Verification items for the finished model (mm, model axes). A direction names the side the tool comes from. Give positions to 0.01 mm unless a question says otherwise; leave off trailing zeros. Order: outer loops, then holes, each group sorted by start corner. A loop starts at its lowest first (then second) coordinate and runs counter-clockwise, first axis right, second up. Notation, with made-up numbers: (14, 73.25) - (19, 73.25) arc R13 cw to (19, 95.25) - close; hole circle Ø10 at (-40, 83). An arc over 180 degrees is marked (long way). Answer as a JSON object with one key per item and string values.
Autodesk Inventor part; units mm, degrees
ref_plane "YZ Plane" through (0, 0, 0) normal (1, 0, 0) x (0, 1, 0)
ref_plane "XZ Plane" through (0, 0, 0) normal (0, 1, 0) x (-1, 0, 0)
ref_plane "XY Plane" through (0, 0, 0) normal (0, 0, 1) x (1, 0, 0)
sketch "Sketch1" plane through (0, 0, 0) normal (0, 1, 0) x (-1, 0, 0)
  arc A0 (0, -16) -> (0, 16) centre (0, 0) ccw
  arc A1 (0, -11.5) -> (0, 11.5) centre (0, 0) ccw
  line L0 (0, 16) -> (0, 11.5)
  line L1 (0, -11.5) -> (0, -16)
  arc A2 (0, -12.5) -> (0, 12.5) centre (0, 0) ccw
  dimension "d0" = 32
  dimension "d1" = 23
  dimension "d2" = 0
  dimension "d3" = 0
  dimension "d4" = 25
  dimension "d5" = 0
  dimension "d6" = 16
  dimension "d7" = 0
  dimension "d8" = 16
extrude "Extrusion1" add sketch "Sketch1" along normal mid plane 4.5 contours L1 A2 L0 A0
extrude "Extrusion2" add sketch "Sketch1" along normal mid plane 1.5 contours L1 A1 L0 A2
sketch "Sketch3" plane through (0, -2.25, -16) normal (1, 0, 0) x (0, 0, -1)
  line L0 (-32, 4.5) -> (-28.5, 4.5)
  line L1 (-30.25, 4.5) -> (-30.25, 4.25)
  line L2 (-28.5, 0) -> (-32, 0)
  line L3 (-30.25, 0) -> (-30.25, 0.25)
  line L4 (-28.5, 3) -> (-28.5, 4.5)
  line L5 (-28.5, 4.25) -> (-32, 4.25)
  line L6 (-33.5, 2.75) -> (-33.5, 1.75)
  line L7 (-32, 0.25) -> (-28.5, 0.25)
  line L8 (-28.5, 0.25) -> (-28.5, 4.25)
  arc A0 (-32, 4.25) -> (-33.5, 2.75) centre (-32, 2.75) ccw
  arc A1 (-33.5, 1.75) -> (-32, 0.25) centre (-32, 1.75) ccw
  circle A2 centre (-30.2, 2.25) radius 1.5
  line L9 (-32, 4.5) -> (-32, 0)
  line L10 (-3.5, 1.5) -> (-28.5, 1.5)
  line L11 (-3.5, 4.25) -> (0, 4.25)
  circle A3 centre (-1.8, 2.25) radius 1.5
  arc A4 (1.5, 2.75) -> (0, 4.25) centre (0, 2.75) ccw
  arc A5 (0, 0.25) -> (1.5, 1.75) centre (0, 1.75) ccw
  line L12 (1.5, 2.75) -> (1.5, 1.75)
  line L13 (-3.5, 3) -> (-3.5, 4.25)
  line L14 (0, 0.25) -> (-3.5, 0.25)
  line L15 (-3.5, 0.25) -> (-3.5, 4.25)
  line L16 (-4.5, 3) -> (-4.5, 1.5)
  line L17 (-27.5, 3) -> (-4.5, 3)
  line L18 (-27.5, 1.5) -> (-27.5, 3)
  line L19 (-4.5, 1.5) -> (-27.5, 1.5)
  point P0 (-16, 2.25)
  dimension "d13" = 3
  dimension "d14" = 5
  dimension "d15" = 2.7
  dimension "d16" = 2.7
  dimension "d17" = 90
  dimension "d18" = 90
  dimension "d19" = 90
  dimension "d20" = 6
  dimension "d21" = 2.75
  dimension "d22" = 1.25
  dimension "d23" = 1
  dimension "d24" = 0
  dimension "d25" = 24
  dimension "d26" = 27.5
  dimension "d27" = 29
  dimension "d28" = 1.5
  dimension "d29" = 3
  dimension "d30" = 25.75
  dimension "d31" = 0.75
  dimension "d32" = 1.5
  dimension "d33" = 1.5
  dimension "d34" = 24
  dimension "d35" = 0.75
  dimension "d36" = 2.75
  dimension "d37" = 1.25
extrude "Extrusion3" add sketch "Sketch3" against normal blind 10 contours L15 L13 L11 A4 L12 A5 L14 | L9 A1 L6 A0 | L5 L4 L8 L7 L9
extrude "Extrusion4" cut sketch "Sketch3" against normal blind 10 contours A2 | A3
properties part number "reverse gear lower trap"
(1) Section check D-D (z = 0). Record the cut outline in (x, y).
Computed values:
{"outline": "(-16, -2.25) - (-12.5, -2.25) - (-12.5, -0.75) - (-11.5, -0.75) - (-11.5, 0.75) - (-12.5, 0.75) - (-12.5, 2.25) - (-16, 2.25) - close"}
(2) Section check A-A (y = 0). Count the separate pieces of the cut face and the enclosed holes in it, then the cut area to 3 significant figures.
Computed values:
{"separate pieces": "3", "enclosed holes": "0", "area": "187 mm²"}
(3) Material ranges on line 1 along Z through (x, y) = (-7.75, 1.05); line 2 along Y through (x, z) = (-6.5, -14.2); line 3 along Z through (x, y) = (-6.75, -0.6), recorded low to high. Write a range as [from, to].
Computed values:
{"line 1": "z = [-17.4, -15.27], [-13.13, -9.81], [9.81, 13.13], [15.27, 17.4]", "line 2": "y = [-2.25, -1.5], [1.5, 2.25]", "line 3": "z = [-17.5, -15.57], [-12.83, -9.31], [9.31, 12.83], [15.57, 17.5]"}
(4) Release check for a two-part mould opening along Z. For faces 4 (the cylindrical face through (-4.93, -1.57, -17.05)), 5 (the cylindrical face through (-12.497, 1.49, 0.275)), 6 (the flat face through (-12, 0.75, 0)), 7 (the flat face through (0, 0, -16)) record: pulls with the +Z half, pulls with the -Z half, needs draft (parallel to the pull), parting line crosses it, or undercut.
Computed values:
{"face 4": "pulls with the -Z half", "face 5": "undercut", "face 6": "undercut", "face 7": "needs draft"}
(5) Access from +Z, -Z, +X, -X, +Y, -Y to the whole of each face (thin tool, end or side, straight path). Record for faces 1 (the flat face through (-10, 0, 16)), 2 (the flat face through (-10, 0, -16)), 3 (the flat face through (-8, 2, -15)).
Computed values:
{"face 1": "+Z, -X, +Y, -Y", "face 2": "-Z, -X, +Y, -Y", "face 3": "-Z, -X, +Y"}
(6) Section check C-C (z = -14.5). Record the cut outline in (x, y), then the cut area to 3 significant figures.
Computed values:
{"outline": "(-10, -2) - (-6.76, -2) - (-6.76, -2.25) - (0, -2.25) - (0, -1.47) - (-10, -1.47) - close; (-10, 1.47) - (0, 1.47) - (0, 2.25) - (-6.76, 2.25) - (-6.76, 2) - (-10, 2) - close", "area": "14.0 mm²"}
